Design review of the part built by this model. Coordinates are the model's own, in mm. Round coordinates to 2 decimals unless told otherwise and drop trailing zeros. Loops run counter-clockwise (first coordinate to the right, second up) from the corner with the lowest first, then second, coordinate; pieces in that order, holes last. Notation, with made-up numbers: M -8.75,-14.5 L 24.25,-14.5 A20 cw 24.25,6.5 Z; hole C 23.5,7 d6. An arc over 180 degrees is marked long. One line per item, written item: value. Start each with the question number.
Item 1: We need section D-D (x = 10.25). Write out the cut boundary in (y, z).
Item 2: We need section C-C (y = 3.75). Write out the cut boundary in (x, z), then the cut area to 3 significant figures.
Item 3: We need section A-A (y = -4). Write out the cut boundary in (x, z).
Item 4: For line 1 along X through (y, z) = (3.75, 0.5); line 2 along X through (y, z) = (-3.5, 0.6); line 3 along X through (y, z) = (3.25, 0.75), list the stretches that pass through material, from the lowest coordinate up.
Item 5: Clearance check with a flat-ended pin moving along its axis: pin 1 (3.5 mm diameter, centred on x = 9.25, y = -4, fed in from +Z). State where the tip first meets the part, or that it passes through.
Item 6: We need section B-B (z = 0.25). State how many separate pieces and enclosed holes the cut face has, then the cut area to 3 significant figures.
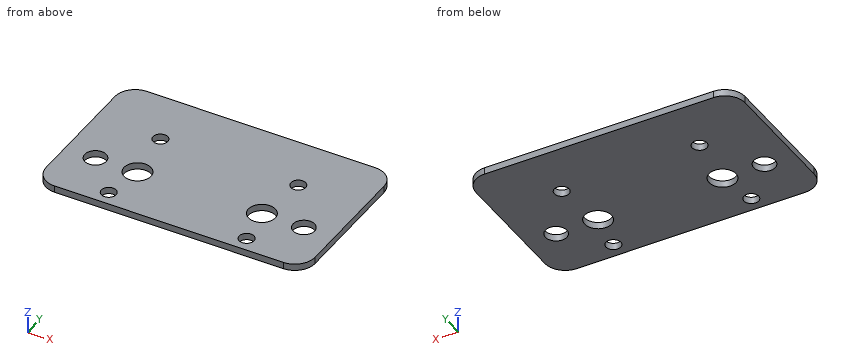
from build123d import *

# Parameters (mm, degrees)
SKETCH1_W           = 40
SKETCH1_H           = 24
SKETCH1_R           = 1.6
BOSS_EXTRUDE1_DEPTH = 1
FILLET1_R           = 3
CUT_EXTRUDE1_DEPTH  = 24.34523506


with BuildPart() as part:
    # Sketch1 → Boss-Extrude1 (new body)
    with BuildSketch(Plane.XY):
        Rectangle(SKETCH1_W, SKETCH1_H)
        with Locations((-15.491933385, -4)):
            Circle(SKETCH1_R, mode=Mode.SUBTRACT)
        with Locations(Location((15.491933385, -4, 0), (0, 0, 180))):
            Circle(SKETCH1_R, mode=Mode.SUBTRACT)
    extrude(amount=BOSS_EXTRUDE1_DEPTH)

    # Fillet1
    fillet1_edges = [part.edges().sort_by_distance(p)[0] for p in [
        (-20, 12, 0.5),
        (20, 12, 0.5),
        (20, -12, 0.5),
        (-20, -12, 0.5),
    ]]
    fillet(fillet1_edges, radius=FILLET1_R)

    # Sketch2 → Cut-Extrude1 (cut, through all)
    with BuildSketch(Plane(origin=(0, 0, 0), x_dir=(-1, 0, 0), z_dir=(0, 0, -1))):
        with BuildLine():
            ThreePointArc((10.25, 4.85), (9.15, 3.75), (10.25, 2.65))
            ThreePointArc((10.25, 2.65), (11.35, 3.75), (10.25, 4.85))
        make_face()
        with BuildLine():
            ThreePointArc((10.25, -8.65), (9.15, -9.75), (10.25, -10.85))
            ThreePointArc((10.25, -10.85), (11.35, -9.75), (10.25, -8.65))
        make_face()
        with BuildLine():
            ThreePointArc((-10.25, 4.85), (-11.35, 3.75), (-10.25, 2.65))
            ThreePointArc((-10.25, 2.65), (-9.15, 3.75), (-10.25, 4.85))
        make_face()
        with BuildLine():
            ThreePointArc((-10.25, -8.65), (-11.35, -9.75), (-10.25, -10.85))
            ThreePointArc((-10.25, -10.85), (-9.15, -9.75), (-10.25, -8.65))
        make_face()
        with BuildLine():
            ThreePointArc((-9.25, -6), (-7.25, -4), (-9.25, -2))
            ThreePointArc((-9.25, -2), (-11.25, -4), (-9.25, -6))
        make_face()
        with BuildLine():
            ThreePointArc((9.25, -2), (7.25, -4), (9.25, -6))
            ThreePointArc((9.25, -6), (11.25, -4), (9.25, -2))
        make_face()
    extrude(amount=-CUT_EXTRUDE1_DEPTH, mode=Mode.SUBTRACT)


solid = part.part
A:
1. outline: M -12,0 L -10.85,0 L -10.85,1 L -12,1 Z; M -8.65,0 L -5.73,0 L -5.73,1 L -8.65,1 Z; M -2.27,0 L 2.65,0 L 2.65,1 L -2.27,1 Z; M 4.85,0 L 12,0 L 12,1 L 4.85,1 Z
2. outline: M -20,0 L -11.35,0 L -11.35,1 L -20,1 Z; M -9.15,0 L 9.15,0 L 9.15,1 L -9.15,1 Z; M 11.35,0 L 20,0 L 20,1 L 11.35,1 Z
2. area: 35.6 mm2
3. outline: M -20,0 L -17.09,0 L -17.09,1 L -20,1 Z; M -13.89,0 L -11.25,0 L -11.25,1 L -13.89,1 Z; M -7.25,0 L 7.25,0 L 7.25,1 L -7.25,1 Z; M 11.25,0 L 13.89,0 L 13.89,1 L 11.25,1 Z; M 17.09,0 L 20,0 L 20,1 L 17.09,1 Z
4. line 1: -20 to -11.35, -9.15 to 9.15, 11.35 to 20
4. line 2: -20 to -17.01, -13.97 to -11.19, -7.31 to 7.31, 11.19 to 13.97, 17.01 to 20
4. line 3: -20 to -11.23, -9.27 to 9.27, 11.23 to 20
5. pin 1: through
6. separate pieces: 1
6. enclosed holes: 8
6. area: 896 mm2
